```python
from build123d import *

# Parameters (mm, degrees)
F0_R          = 11.5
F1_DEPTH      = 820
F2_R          = 6.5
F3_DEPTH      = 100
F3_DEPTH_BACK = 25


with BuildPart() as f1:
    # F0 (on Top) → F1 (new body)
    with BuildSketch(Plane.XY):
        Circle(F0_R)
    extrude(amount=F1_DEPTH)

    # F2 (on Right) → F3 (cut, two sides)
    with BuildSketch(Plane.YZ) as f3_sk:
        with Locations((0, 27)):
            Circle(F2_R)
        with Locations((0, 93)):
            Circle(F2_R)
    extrude(amount=-F3_DEPTH, mode=Mode.SUBTRACT)
    extrude(f3_sk.sketch, amount=F3_DEPTH_BACK, mode=Mode.SUBTRACT)


solid = f1.part
```
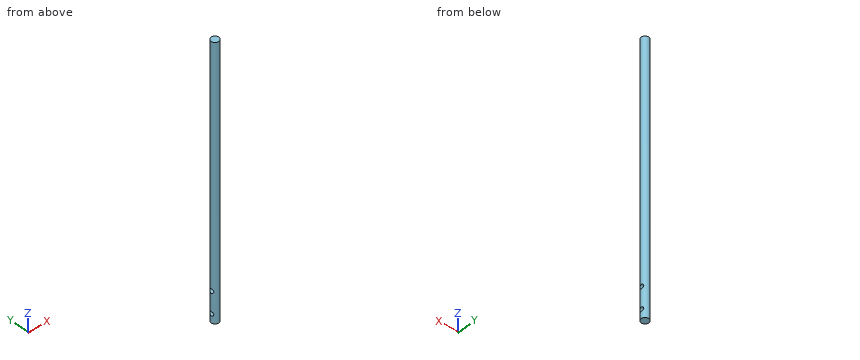
Geometry check sheet. Reference: the model listing, model coordinates, mm. Coordinates: 2 decimals unless noted, no trailing zeros. Loops run counter-clockwise (first coordinate to the right, second up) from the corner with the lowest first, then second, coordinate; pieces in that order, holes last. Notation, with made-up numbers: (22.25, -9.75) -> (45.25, -9.75) arc R28 ccw to (45.25, 11.25) -> close; hole circle Ø2 at (89.5, 15.5). An arc over 180 degrees is marked (long way). Put each result on its own line as item: value.
1) Cross-section at A-A on y = 0. Record the boundary of the cut face in (x, z).
Result set:
outline: (-11.5, 0) -> (11.5, 0) -> (11.5, 20.5) -> (-11.5, 20.5) -> close; (-11.5, 33.5) -> (11.5, 33.5) -> (11.5, 86.5) -> (-11.5, 86.5) -> close; (-11.5, 99.5) -> (11.5, 99.5) -> (11.5, 820) -> (-11.5, 820) -> close
2) Cross-section at B-B on z = 259. Record the boundary of the cut face in (x, y), plus the area to 3 significant figures.
Result set:
outline: circle Ø23 at (0, 0)
area: 415 mm^2
3) Thickness scan on line 1 (Z direction, x = -2.5, y = 0); line 2 (Z direction, x = 7.25, y = -1.25); line 3 (Y direction, x = -0.75, z = 772). Record the ranges inside material, lowest first.
Result set:
line 1: z = 0 to 20.5, 33.5 to 86.5, 99.5 to 820
line 2: z = 0 to 20.62, 33.38 to 86.62, 99.38 to 820
line 3: y = -11.48 to 11.48
4) Gauge pin test, flat ends, axial feed: pin 1 Ø10 at (x, z) = (-9, 248) entering from -Y; pin 2 Ø12 at (x, z) = (-5, 268.5) entering from -Y; pin 3 Ø11.5 at (y, z) = (0, 27) entering from +X; pin 4 Ø6 at (y, z) = (-4, 390) entering from +X. Record the tip position at first contact, or that the pin passes through.
Result set:
pin 1: stops at y = -10.78
pin 2: stops at y = -11.5
pin 3: passes through
pin 4: stops at x = 11.46
